from build123d import *

# Parameters (mm, degrees)
BLANKSKE_W         = 61
BLANKSKE_H         = 14.5
BLANK_DEPTH        = 6.5
TOOTHCUTSIM_DEPTH  = 64.035704168
TEETHCUTS_COUNT    = 14
TEETHCUTS_PITCH    = 4.712388975
CUT_EXTRUDE1_DEPTH = 6.5


with BuildPart() as part:
    # BlankSke → Blank (new body)
    with BuildSketch(Plane.XY):
        with Locations((30.5, 7.25)):
            Rectangle(BLANKSKE_W, BLANKSKE_H)
    extrude(amount=-BLANK_DEPTH)

    # TooCutSkeSim → ToothCutSim (cut, through all)
    with BuildSketch(Plane.XY):
        Polygon((0.654653055, 11.125), (-0.654653055, 11.125), (-1.892297439, 14.5254), (1.892297439, 14.5254), align=None)
    toothcutsim = extrude(amount=-TOOTHCUTSIM_DEPTH, mode=Mode.SUBTRACT)

    # TeethCuts: ToothCutSim ×14
    with Locations(*[(i * TEETHCUTS_PITCH, 0, 0) for i in range(1, TEETHCUTS_COUNT)]):
        add(toothcutsim, mode=Mode.SUBTRACT)

    # Sketch1 → Cut-Extrude1 (cut)
    with BuildSketch(Plane(origin=(0, 0, -6.5), x_dir=(-1, 0, 0), z_dir=(0, 0, -1))):
        with BuildLine():
            Line((-44, 8.125), (-54, 8.125))
            ThreePointArc((-54, 8.125), (-55.81827458, 6.957993128), (-55.51461023, 4.818877551))
            Line((-55.51461023, 4.818877551), (-52.48538977, 1.306122449))
            ThreePointArc((-52.48538977, 1.306122449), (-52.125270625, 0.696699196), (-52, 0))
            Line((-52, 0), (-46, 0))
            ThreePointArc((-46, 0), (-45.874729375, 0.696699196), (-45.51461023, 1.306122449))
            Line((-45.51461023, 1.306122449), (-42.48538977, 4.818877551))
            ThreePointArc((-42.48538977, 4.818877551), (-42.18172542, 6.957993128), (-44, 8.125))
        make_face()
    extrude(amount=-CUT_EXTRUDE1_DEPTH, mode=Mode.SUBTRACT)


solid = part.part
Source: CAD feature listing. Evaluate the final solid. Frame: model axes, mm. A direction names the side the tool comes from. Give positions to 0.01 mm unless a question says otherwise; leave off trailing zeros. Order: outer loops, then holes, each group sorted by start corner. A loop starts at its lowest first (then second) coordinate and runs counter-clockwise, first axis right, second up. Notation, with made-up numbers: (-13, 62) -> (-3, 62) arc R25 ccw to (-3, 94) -> close; hole circle Ø6 at (45.5, 59). An arc over 180 degrees is marked (long way). Write item = value, one per line.
Q1. Pull-direction query (Y, two-part tool) for faces 3 (the face through (54.021, 3.087, -3.296)), 4 (the face through (34.264, 12.836, -3.204)), 5 (the face through (56, 0, -3)); classes: released by +Y, released by -Y, zero draft, split by the parting line, or undercut.
Data:
face_3 = undercut
face_4 = released by +Y
face_5 = released by -Y
Q2. Set-up query: faces 1 (the face through (2.3, 14.5, -3.2)), 2 (the face through (22.3, 12.79, -3.2)). Return all of +Z, -Z, +X, -X, +Y, -Y with unobstructed straight access to the full face (end or side cutting, diameter ignored); none if empty.
Data:
face_1 = +Z, -Z, +X, -X, +Y
face_2 = +Z, -Z, +Y
Q3. Material intervals for line 1 (X direction, y = 6, z = -1.5); line 2 (X direction, y = 2.75, z = -1); line 3 (Y direction, x = 14, z = -2) (3 decimals), sorted ascending. Write a range as from..to.
Data:
line_1 = 0..42, 56..61
line_2 = 0..44.27, 53.73..61
line_3 = 0..11.125
Q4. Pin query (flat end, axial travel): pin 1 (0.7 mm diameter, centred on x = 4.5, z = -3.5, fed in from +Y) (3 decimals). Return the tip coordinate at first contact, or that it passes through.
Data:
pin_1 = 11.125
Q5. Cut plane D-D, the plane y = 13.5. State how many separate pieces and enclosed holes the cut face has, and give its area (3 significant figures).
Data:
separate_pieces = 13
enclosed_holes = 0
area = 141 mm^2
Q6. Cut plane C-C, the plane x = 23.5. Output: boundary loops of the cut face in (y, z) (3 decimals), and give its area (3 significant figures).
Data:
outline = (0, -6.5) -> (11.125, -6.5) -> (11.125, 0) -> (0, 0) -> close
area = 72.3 mm^2
Q7. Cut plane A-A, the plane y = 2.5. Output: boundary loops of the cut face in (x, z), and give its area (3 significant figures).
Data:
outline = (0, -6.5) -> (44.49, -6.5) -> (44.49, 0) -> (0, 0) -> close; (53.51, -6.5) -> (61, -6.5) -> (61, 0) -> (53.51, 0) -> close
area = 338 mm^2
Q8. Cut plane B-B, the plane x = 53. Output: boundary loops of the cut face in (y, z) (3 decimals), and give its area (3 significant figures).
Data:
outline = (0, -6.5) -> (1.903, -6.5) -> (1.903, 0) -> (0, 0) -> close; (8.125, -6.5) -> (12.524, -6.5) -> (12.524, 0) -> (8.125, 0) -> close
area = 41.0 mm^2
